```python
from build123d import *

# Parameters (mm, degrees)
SKETCH1_W           = 13.6
SKETCH1_H           = 13.6
BOSS_EXTRUDE1_DEPTH = 5
SKETCH2_R           = 6.1
CUT_EXTRUDE1_DEPTH  = 3.2
SKETCH3_W           = 13.6
SKETCH3_H           = 5
BOSS_EXTRUDE2_DEPTH = 63.5
FILLET1_R           = 0.2
FILLET2_R           = 9
SKETCH10_W          = 27.6
SKETCH10_H          = 6
BOSS_EXTRUDE5_DEPTH = 7
SKETCH11_R          = 1.75
CUT_EXTRUDE4_DEPTH  = 67.220314104
FILLET3_R           = 10
FILLET4_R           = 3.5
FILLET5_R           = 1


# Some blends are built 0.0001 mm under size
with BuildPart() as part:
    # Sketch1 → Boss-Extrude1 (new body)
    with BuildSketch(Plane(origin=(0, 0, 0), x_dir=(1, 0, 0), z_dir=(0, 1, 0))):
        Rectangle(SKETCH1_W, SKETCH1_H)
    extrude(amount=BOSS_EXTRUDE1_DEPTH)

    # Sketch2 → Cut-Extrude1 (cut)
    with BuildSketch(Plane(origin=(0, 5, 0), x_dir=(1, 0, 0), z_dir=(0, 1, 0))):
        with Locations(Location((0, 0, 0), (0, 0, 270))):
            Circle(SKETCH2_R)
    extrude(amount=-CUT_EXTRUDE1_DEPTH, mode=Mode.SUBTRACT)

    # Sketch3 → Boss-Extrude2 (add)
    with BuildSketch(Plane.XZ):
        with Locations((0, 4.3)):
            Rectangle(SKETCH3_W, SKETCH3_H)
    extrude(amount=BOSS_EXTRUDE2_DEPTH)

    # Fillet1
    fillet1_edges = [part.edges().sort_by_distance(p)[0] for p in [
        (0, 5, -6.1),
    ]]
    fillet(fillet1_edges, radius=FILLET1_R)

    # Fillet2
    # the kernel refuses this fillet: 9 mm, written as the material it adds along each edge
    with BuildSketch(Plane(origin=(6.8, 0, 1.8), x_dir=(0, 0, -1), z_dir=(-1, 0, 0))) as fillet2_piece_1:
        with BuildLine():
            CenterArc((9, 8.991106717), FILLET2_R, 180, 87.452681817)
            Line((0, 8.991106717), (-0.18, 8.991106717))
            Line((-0.18, 8.991106717), (-0.18, 0))
            Line((-0.18, 0), (0, -0.18))
            ThreePointArc((0, -0.18), (4.3, -0.18), (8.592, -0.179822134))
            Line((8.592, -0.179822134), (8.6, 0))
        make_face()
    extrude(amount=13.6)

    # Sketch10 → Boss-Extrude5 (add)
    with BuildSketch(Plane(origin=(0, 0, 1.8), x_dir=(-1, 0, 0), z_dir=(0, 0, -1))):
        with Locations((7, -60.5)):
            Rectangle(SKETCH10_W, SKETCH10_H)
    extrude(amount=BOSS_EXTRUDE5_DEPTH)

    # Sketch11 → Cut-Extrude4 (cut, through all)
    with BuildSketch(Plane(origin=(0, -57.5, 0), x_dir=(1, 0, 0), z_dir=(0, 1, 0))):
        with Locations(Location((-10.3, 1.7, 0), (0, 0, 270))):
            Circle(SKETCH11_R)
        with Locations(Location((-17.3, 1.7, 0), (0, 0, 270))):
            Circle(SKETCH11_R)
    extrude(amount=-CUT_EXTRUDE4_DEPTH, mode=Mode.SUBTRACT)

    # Fillet3
    # the kernel refuses this fillet: 10 mm, written as the material it adds along each edge
    with BuildSketch(Plane(origin=(-6.8, -57.5, 1.8), x_dir=(0, 0, 1), z_dir=(0, -1, 0))) as fillet3_piece_1:
        with BuildLine():
            CenterArc((10, 8.660254038), FILLET3_R, 180, 60)
            Line((0, 8.660254038), (0, 0))
            Line((0, 0), (5, 0))
        make_face()
    extrude(amount=6)

    # Fillet4
    fillet4_edges = [part.edges().sort_by_distance(p)[0] for p in [
        (-20.8, -60.5, 1.8),
        (-20.8, -60.5, -5.2),
        (6.8, -60.5, -5.2),
    ]]
    fillet(fillet4_edges, radius=FILLET4_R - 0.0001)  # a hair under: the kernel refuses the full size

    # Fillet5
    fillet5_edges = [part.edges().sort_by_distance(p)[0] for p in [
        (0, -57.5, 1.8),
        (-6.8, -57.5, 4.3),
    ]]
    fillet(fillet5_edges, radius=FILLET5_R)


solid = part.part
```
Check sheet for the modelled part. Datum: model origin and axes. Units: mm. A direction names the side the tool comes from. Round coordinates to 2 decimals unless told otherwise and drop trailing zeros. Loops run counter-clockwise (first coordinate to the right, second up) from the corner with the lowest first, then second, coordinate; pieces in that order, holes last. Notation, with made-up numbers: (27.5, 22) - (51.5, 22) arc R21 ccw to (51.5, 32) - close; hole circle Ø3 at (89.5, 82). An arc over 180 degrees is marked (long way). Answer as a JSON object with one key per item and string values. Group by question number.
Q1. Sectioned sample at B-B, the plane y = -39. Enter the section's corners in (x, z).
Q2. Gauge pin test, flat ends, axial feed: P1, Ø2, axis at y = -19, z = 4.5, coming from the -X side; P2, Ø11, axis at x = 1.5, y = -27.5, coming from the -Z side; P3, Ø5, axis at x = -9.5, y = -31, coming from the -Z side. Record the tip position at first contact, or that the pin passes through.
Q3. Mould release check, pull along X, two halves, no side actions. Record for faces 1 (the face through (5.8, -60.46, -4.15)), 2 (the face through (0, 2, -6.8)), 3 (the face through (-10.22, -60.46, -3.45)): released by +X, released by -X, zero draft, split by the parting line, or undercut.
Q4. Set-up check for faces 4 (the face through (0.1, -2.84, -0.63)), 5 (the face through (-6.8, -19, 3)), 6 (the face through (-7, -60, -5.2)), 7 (the face through (-3.71, 3.32, -4.84)): record each of +Z, -Z, +X, -X, +Y, -Y from which the full face is reachable in a straight line by a thin tool's end or side.
Solution:
{
 "1": {"outline": "(-6.8, 1.8) - (6.8, 1.8) - (6.8, 6.8) - (-6.8, 6.8) - close"},
 "2": {"P1": "stops at x = -6.8", "P2": "stops at z = 1.8", "P3": "passes through"},
 "3": {"face 1": "released by +X", "face 2": "zero draft", "face 3": "undercut"},
 "4": {"face 4": "-Z, +X, -X", "face 5": "+Z, -Z, -X, +Y", "face 6": "-Z, +X, -X, -Y", "face 7": "+Y"}
}
